The model under review builds one solid part; all positions refer to its coordinate system, in mm. Face numbers are marked on the shaded views. Round coordinates to 2 decimals unless told otherwise and drop trailing zeros. Order: outer loops, then holes, each group sorted by start corner. A loop starts at its lowest first (then second) coordinate and runs counter-clockwise, first axis right, second up. Notation, with made-up numbers: M 57.5,67.25 L 86.5,67.25 A18 ccw 86.5,101.25 Z; hole C -7.5,-29.75 d1. An arc over 180 degrees is marked long. Use a Markdown table: item, result. Add a question column.
1. Consider section C-C on z = -18. State the section outline as (x, y) points, then the cut area to 3 significant figures.
2. Consider section B-B on x = 26. State the section outline as (y, z) points, then the cut area to 3 significant figures.
3. Consider section D-D on y = -0.25. State the section outline as (x, z) points.
4. Consider section A-A on y = -6. State the section outline as (x, z) points.
5. The part is to be moulded in two halves that separate along X. For the marked faces 1, 2 and 3, say which applies: +X half, -X half, draft (parallel to the pull), parting line (faces both ways), or undercut.
6. To check wall thickness, follow probe 1 along X at (y, z) = (-0.75, -21); probe 2 along X at (y, z) = (-0.75, -28); probe 3 along Z at (x, y) = (18.5, -6.25). State the ranges of each line that lie inside material, in increasing order.
7. Insertion check: P1, Ø2, axis at x = 29, z = -29, coming from the -Y side; P2, Ø1.6, axis at x = 33.5, y = -1, coming from the +Z side; P3, Ø1.6, axis at y = -1, z = -18.5, coming from the +X side. Each pin has a flat end and moves straight along its axis. Give the tip position at first contact, or say it passes through.
from build123d import *

# Parameters (mm, degrees)
F1_DEPTH       = 7
F3_D           = 3.3
F3_CSINK_D     = 6.72
F3_CSINK_ANGLE = 90
F4_DEPTH       = 1.5


with BuildPart() as f1:
    # F0 (on Front) → F1 (new body)
    with BuildSketch(Plane.XZ):
        with BuildLine():
            ThreePointArc((20.6767564522, -31.0453001757), (23.505183577, -29.8737273005), (24.6767564522, -27.0453001757))
            ThreePointArc((24.6767564522, -27.0453001757), (23.505183577, -24.216873051), (20.6767564522, -23.0453001757))
            ThreePointArc((20.6767564522, -23.0453001757), (17.8483293275, -24.216873051), (16.6767564522, -27.0453001757))
            ThreePointArc((16.6767564522, -27.0453001757), (17.8483293275, -29.8737273005), (20.6767564522, -31.0453001757))
        make_face()
    extrude(amount=F1_DEPTH)

    # F3 (through all)
    with Locations(Plane(origin=(0, 0, 0), x_dir=(1, 0, 0), z_dir=(0, 1, 0))):
        with Locations((20.6767564522, 27.0453001757)):
            CounterSinkHole(F3_D / 2, F3_CSINK_D / 2, counter_sink_angle=F3_CSINK_ANGLE)

    # F0 (on Front) → F4 (join)
    with BuildSketch(Plane.XZ):
        with BuildLine():
            ThreePointArc((16.6767564522, -27.0453001757), (17.8483293275, -24.216873051), (20.6767564522, -23.0453001757))
            Line((20.6767564522, -23.0453001757), (20.6767564522, -14.3548102902))
            Line((20.6767564522, -14.3548102902), (16.6767564522, -14.3548102902))
            Line((16.6767564522, -14.3548102902), (16.6767564522, -27.0453001757))
        make_face()
        with BuildLine():
            Line((37.8486532164, -27.0453001757), (24.6767564522, -27.0453001757))
            ThreePointArc((24.6767564522, -27.0453001757), (23.505183577, -29.8737273005), (20.6767564522, -31.0453001757))
            Line((20.6767564522, -31.0453001757), (37.8486532164, -31.0453001757))
            Line((37.8486532164, -31.0453001757), (37.8486532164, -27.0453001757))
        make_face()
    extrude(amount=F4_DEPTH)


solid = f1.part
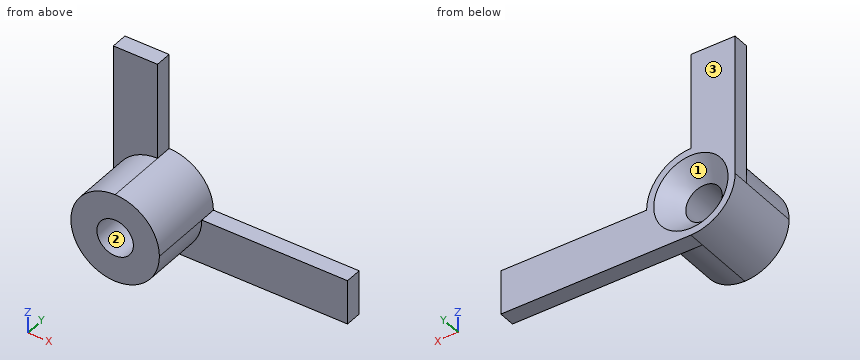
Answer block:
| question | item | result |
|---|---|---|
| 1 | outline | M 16.68,-1.5 L 20.68,-1.5 L 20.68,0 L 16.68,0 Z |
| 1 | area | 6.00 mm^2 |
| 2 | outline | M -1.5,-31.05 L 0,-31.05 L 0,-27.05 L -1.5,-27.05 Z |
| 2 | area | 6.00 mm^2 |
| 3 | outline | M 16.68,-27.05 A4 ccw 20.68,-31.05 L 37.85,-31.05 L 37.85,-27.05 L 24.68,-27.05 A4 ccw 20.68,-23.05 L 20.68,-14.35 L 16.68,-14.35 Z; hole C 20.68,-27.05 d6.22 |
| 4 | outline | C 20.68,-27.05 d8; hole C 20.68,-27.05 d3.3 |
| 5 | face 1 | undercut |
| 5 | face 2 | undercut |
| 5 | face 3 | draft |
| 6 | probe 1 | 16.68 to 20.68 |
| 6 | probe 2 | 16.79 to 18.25, 23.11 to 37.85 |
| 6 | probe 3 | -30.4 to -23.69 |
| 7 | P1 | y = -1.5 |
| 7 | P2 | z = -27.05 |
| 7 | P3 | x = 20.68 |
